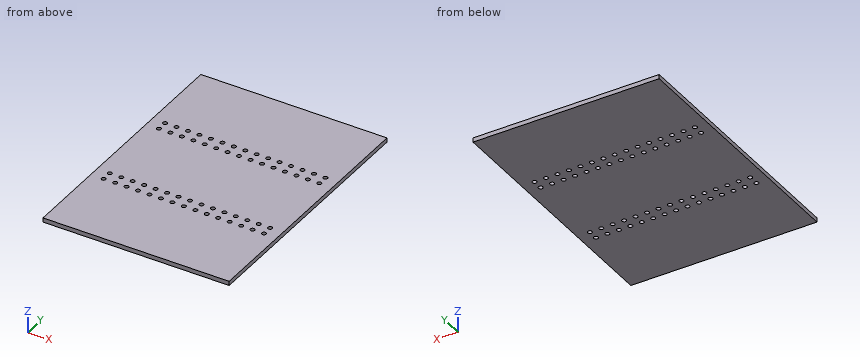
```python
from build123d import *

# Parameters (mm, degrees)
F0_W     = 130
F0_H     = 180
F0_R     = 1.5
F1_DEPTH = 3


with BuildPart() as f1:
    # F0 (on Top) → F1 (new body)
    with BuildSketch(Plane.XY):
        with Locations((-81.050769, 20.358638)):
            Rectangle(F0_W, F0_H)
        with Locations((-137.050769, -15.141362)):
            Circle(F0_R, mode=Mode.SUBTRACT)
        with Locations((-129.050769, -15.141362)):
            Circle(F0_R, mode=Mode.SUBTRACT)
        with Locations((-121.050769, -15.141362)):
            Circle(F0_R, mode=Mode.SUBTRACT)
        with Locations((-113.050769, -15.141362)):
            Circle(F0_R, mode=Mode.SUBTRACT)
        with Locations((-137.050769, -8.141362)):
            Circle(F0_R, mode=Mode.SUBTRACT)
        with Locations((-129.050769, -8.141362)):
            Circle(F0_R, mode=Mode.SUBTRACT)
        with Locations((-121.050769, -8.141362)):
            Circle(F0_R, mode=Mode.SUBTRACT)
        with Locations((-113.050769, -8.141362)):
            Circle(F0_R, mode=Mode.SUBTRACT)
        with Locations((-105.050769, -15.141362)):
            Circle(F0_R, mode=Mode.SUBTRACT)
        with Locations((-97.050769, -15.141362)):
            Circle(F0_R, mode=Mode.SUBTRACT)
        with Locations((-89.050769, -15.141362)):
            Circle(F0_R, mode=Mode.SUBTRACT)
        with Locations((-81.050769, -15.141362)):
            Circle(F0_R, mode=Mode.SUBTRACT)
        with Locations((-105.050769, -8.141362)):
            Circle(F0_R, mode=Mode.SUBTRACT)
        with Locations((-97.050769, -8.141362)):
            Circle(F0_R, mode=Mode.SUBTRACT)
        with Locations((-89.050769, -8.141362)):
            Circle(F0_R, mode=Mode.SUBTRACT)
        with Locations((-81.050769, -8.141362)):
            Circle(F0_R, mode=Mode.SUBTRACT)
        with Locations((-73.050769, -15.141362)):
            Circle(F0_R, mode=Mode.SUBTRACT)
        with Locations((-65.050769, -15.141362)):
            Circle(F0_R, mode=Mode.SUBTRACT)
        with Locations((-57.050769, -15.141362)):
            Circle(F0_R, mode=Mode.SUBTRACT)
        with Locations((-49.050769, -15.141362)):
            Circle(F0_R, mode=Mode.SUBTRACT)
        with Locations((-41.050769, -15.141362)):
            Circle(F0_R, mode=Mode.SUBTRACT)
        with Locations((-73.050769, -8.141362)):
            Circle(F0_R, mode=Mode.SUBTRACT)
        with Locations((-65.050769, -8.141362)):
            Circle(F0_R, mode=Mode.SUBTRACT)
        with Locations((-57.050769, -8.141362)):
            Circle(F0_R, mode=Mode.SUBTRACT)
        with Locations((-49.050769, -8.141362)):
            Circle(F0_R, mode=Mode.SUBTRACT)
        with Locations((-41.050769, -8.141362)):
            Circle(F0_R, mode=Mode.SUBTRACT)
        with Locations((-33.050769, -15.141362)):
            Circle(F0_R, mode=Mode.SUBTRACT)
        with Locations((-25.050769, -15.141362)):
            Circle(F0_R, mode=Mode.SUBTRACT)
        with Locations((-33.050769, -8.141362)):
            Circle(F0_R, mode=Mode.SUBTRACT)
        with Locations((-25.050769, -8.141362)):
            Circle(F0_R, mode=Mode.SUBTRACT)
        with Locations((-137.050769, 47.858638)):
            Circle(F0_R, mode=Mode.SUBTRACT)
        with Locations((-129.050769, 47.858638)):
            Circle(F0_R, mode=Mode.SUBTRACT)
        with Locations((-121.050769, 47.858638)):
            Circle(F0_R, mode=Mode.SUBTRACT)
        with Locations((-113.050769, 47.858638)):
            Circle(F0_R, mode=Mode.SUBTRACT)
        with Locations((-137.050769, 54.858638)):
            Circle(F0_R, mode=Mode.SUBTRACT)
        with Locations((-129.050769, 54.858638)):
            Circle(F0_R, mode=Mode.SUBTRACT)
        with Locations((-121.050769, 54.858638)):
            Circle(F0_R, mode=Mode.SUBTRACT)
        with Locations((-113.050769, 54.858638)):
            Circle(F0_R, mode=Mode.SUBTRACT)
        with Locations((-105.050769, 47.858638)):
            Circle(F0_R, mode=Mode.SUBTRACT)
        with Locations((-97.050769, 47.858638)):
            Circle(F0_R, mode=Mode.SUBTRACT)
        with Locations((-89.050769, 47.858638)):
            Circle(F0_R, mode=Mode.SUBTRACT)
        with Locations((-81.050769, 47.858638)):
            Circle(F0_R, mode=Mode.SUBTRACT)
        with Locations((-105.050769, 54.858638)):
            Circle(F0_R, mode=Mode.SUBTRACT)
        with Locations((-97.050769, 54.858638)):
            Circle(F0_R, mode=Mode.SUBTRACT)
        with Locations((-89.050769, 54.858638)):
            Circle(F0_R, mode=Mode.SUBTRACT)
        with Locations((-81.050769, 54.858638)):
            Circle(F0_R, mode=Mode.SUBTRACT)
        with Locations((-73.050769, 47.858638)):
            Circle(F0_R, mode=Mode.SUBTRACT)
        with Locations((-65.050769, 47.858638)):
            Circle(F0_R, mode=Mode.SUBTRACT)
        with Locations((-57.050769, 47.858638)):
            Circle(F0_R, mode=Mode.SUBTRACT)
        with Locations((-49.050769, 47.858638)):
            Circle(F0_R, mode=Mode.SUBTRACT)
        with Locations((-41.050769, 47.858638)):
            Circle(F0_R, mode=Mode.SUBTRACT)
        with Locations((-73.050769, 54.858638)):
            Circle(F0_R, mode=Mode.SUBTRACT)
        with Locations((-65.050769, 54.858638)):
            Circle(F0_R, mode=Mode.SUBTRACT)
        with Locations((-57.050769, 54.858638)):
            Circle(F0_R, mode=Mode.SUBTRACT)
        with Locations((-49.050769, 54.858638)):
            Circle(F0_R, mode=Mode.SUBTRACT)
        with Locations((-41.050769, 54.858638)):
            Circle(F0_R, mode=Mode.SUBTRACT)
        with Locations((-33.050769, 47.858638)):
            Circle(F0_R, mode=Mode.SUBTRACT)
        with Locations((-25.050769, 47.858638)):
            Circle(F0_R, mode=Mode.SUBTRACT)
        with Locations((-33.050769, 54.858638)):
            Circle(F0_R, mode=Mode.SUBTRACT)
        with Locations((-25.050769, 54.858638)):
            Circle(F0_R, mode=Mode.SUBTRACT)
    extrude(amount=F1_DEPTH)


solid = f1.part
```
Design review of the part built by this model. Coordinates are the model's own, in mm. Coordinates: 2 decimals unless noted, no trailing zeros. One line per question, with ' | ' between items.
(1) For pin 1 Ø2.5 at (x, y) = (-137.05, -8.14) entering from +Z; pin 2 Ø4 at (x, y) = (-25.05, -15.14) entering from -Z, all flat-tipped, find the tip position at first contact; note any pin that passes through.
Filled in:
pin 1: passes through | pin 2: stops at z = 0
(2) We need section A-A (z = 1.15). Count the separate pieces of the cut face and the enclosed holes in it, and give its area (3 significant figures).
Filled in:
separate pieces: 1 | enclosed holes: 60 | area: 23,000 mm^2
(3) Wall thickness on probe 1 along Y at (x, z) = (-57, 2.45); probe 2 along Y at (x, z) = (-32, 2.4): over which ranges is each line inside the solid? List them lowest first.
Filled in:
probe 1: y = -69.64 to -16.64, -13.64 to -9.64, -6.64 to 46.36, 49.36 to 53.36, 56.36 to 110.36 | probe 2: y = -69.64 to -16.21, -14.07 to -9.21, -7.07 to 46.79, 48.93 to 53.79, 55.93 to 110.36
